Geometry check sheet. Reference: the model listing, model coordinates, mm. Face numbers are marked on the shaded views. Give positions to 0.01 mm unless a question says otherwise; leave off trailing zeros. Loops run counter-clockwise (first coordinate to the right, second up) from the corner with the lowest first, then second, coordinate; pieces in that order, holes last. Notation, with made-up numbers: (-9, 12.25) -> (42, 12.25) arc R22 cw to (42, 47.25) -> close; hole circle Ø6 at (-7.75, 54). An arc over 180 degrees is marked (long way). Answer in a Markdown table with one row per item. Add a question column.
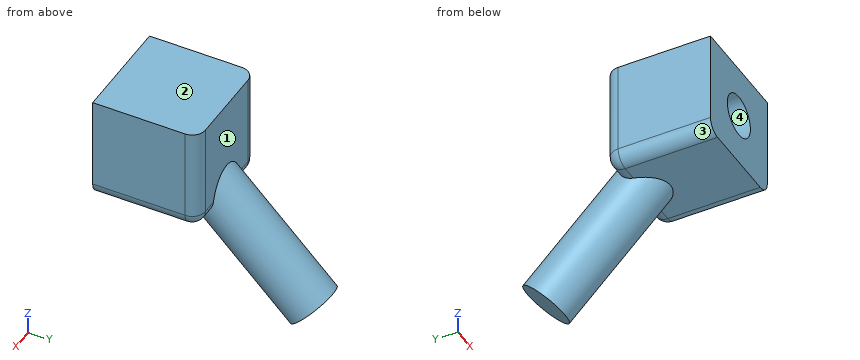
Autodesk Inventor part; units mm, degrees
ref_plane "Work Plane3" through (0, 8, 8) normal (0, -0.7071068, 0.7071068) x (-1, 0, 0)
ref_plane "YZ Plane" through (0, 0, 0) normal (1, 0, 0) x (0, 1, 0)
ref_plane "XZ Plane" through (0, 0, 0) normal (0, 1, 0) x (-1, 0, 0)
sketch "Sketch1" plane through (0, 0, 0) normal (0, 0, 1) x (1, 0, 0)
  line L0 (-8, 8) -> (0, 8)
  line L1 (0, 8) -> (0, 0)
  line L2 (0, 0) -> (-8, 0)
  line L3 (-8, 0) -> (-8, 8)
  dimension "d0" = 8
  dimension "d1" = 8
extrude "Extrusion1" add sketch "Sketch1" along normal blind 8
sketch "Sketch5" plane through (0, 0, 8) normal (0, 0, 1) x (1, 0, 0)
  point P0 (0, 0)
sketch "Sketch8" plane through (-8, 8, 0) normal (0, 1, 0) x (1, 0, 0)
  line L0 (8, -8) -> (0, -8)
  line L1 (0, 0) -> (0, -8)
  point P0 (8, 0)
  point P1 (4, -3)
  dimension "d14" = 5
  dimension "d15" = 4
ref_plane "Work Plane3" through (0, 8, 8) normal (0, -0.7071068, 0.7071068) x (-1, 0, 0)
sketch "Sketch11" plane through (0, 8, 8) normal (0, -0.7071068, 0.7071068) x (-1, 0, 0)
  line L0 (8, 5.6569) -> (0, 5.6569)
  circle A0 centre (4, 5.6569) radius 2
  point P0 (0, 11.3137)
  dimension "d21" = 4
extrude "Extrusion4" add sketch "Sketch11" against normal blind 15
sketch "Sketch12" plane through (-8, 0, 0) normal (0, -1, 0) x (1, 0, 0)
  point P0 (8, 0)
  point P1 (4, 4)
  dimension "d24" = 4
  dimension "d25" = 4
hole "Hole1" at (-4, 0, 4) direction (0, 1, 0) diameter 3.242 depth 5 tip angle 118
fillet "Fillet1" radius 1 6 edges at (-7, 8, 0) (-8, 8, 4) (-8, 4, 0) (-1, 8, 0) (0, 8, 4) (0, 4, 0)
properties part number "as2"
1. Material ranges on L1, parallel to X at y = 3.05, z = 4; L2, parallel to Z at x = -4, y = 2.6; L3, parallel to Y at x = -6.5, z = 1, recorded low to high. Write a range as from..to.
2. Sectioned sample at A-A (y = 4.75). Enter the section's corners in (x, z), plus the area to 3 significant figures.
3. Sectioned sample at B-B (x = -1.25). Enter the section's corners in (y, z).
4. Release check for a two-part mould opening along Z. For the marked faces 1, 2, 3 and 4 record: released by +Z, released by -Z, zero draft, split by the parting line, or undercut.
5. Gauge pin test, flat ends, axial feed: pin 1 Ø3 at (x, z) = (-4, 4) entering from -Y; pin 2 Ø4 at (y, z) = (12, 1) entering from -X; pin 3 Ø3 at (x, z) = (-3.5, 3) entering from +Y. Record the tip position at first contact, or that the pin passes through.
Response:
| question | item | result |
|---|---|---|
| 1 | L1 | x = -8..-5.62, -2.38..0 |
| 1 | L2 | z = 0..2.38, 5.62..8 |
| 1 | L3 | y = 0..8 |
| 2 | outline | (-8, 1) arc R1 ccw to (-7, 0) -> (-1, 0) arc R1 ccw to (0, 1) -> (0, 8) -> (-8, 8) -> close; hole circle Ø3.24 at (-4, 4) |
| 2 | area | 55.3 mm2 |
| 3 | outline | (0, 0) -> (7, 0) arc R1 ccw to (8, 1) -> (8, 8) -> (0, 8) -> close |
| 4 | face 1 | zero draft |
| 4 | face 2 | released by +Z |
| 4 | face 3 | released by -Z |
| 4 | face 4 | undercut |
| 5 | pin 1 | stops at y = 5.07 |
| 5 | pin 2 | stops at x = -5.28 |
| 5 | pin 3 | stops at y = 9.29 |
